Read the model definition and answer for the solid it produces. Units are mm, in the model's axes. A direction names the side the tool comes from. Coordinates: 2 decimals unless noted, no trailing zeros. Loops run counter-clockwise (first coordinate to the right, second up) from the corner with the lowest first, then second, coordinate; pieces in that order, holes last.
from build123d import *

# Parameters (mm, degrees)
PAD_DEPTH       = 8
SKETCH001_R     = 5.2
SKETCH001_R_2   = 1.75
POCKET_DEPTH    = 8.001
SKETCH002_W     = 60
SKETCH002_H     = 8
PAD001_DEPTH    = 14
SKETCH003_R     = 2.8
POCKET001_DEPTH = 30.001
FILLET_R        = 23
FILLET001_R     = 5
CHAMFER_SIZE    = 1
FILLET002_R     = 2


with BuildPart() as part:
    # Sketch → Pad (new body)
    with BuildSketch(Plane.XY):
        Polygon((-30, 0), (-30, 10), (-10, 30), (10, 30), (30, 10), (30, 0), align=None)
    extrude(amount=PAD_DEPTH)

    # Sketch001 → Pocket (cut, through all)
    with BuildSketch(Plane.XY.offset(8)):
        with Locations((0, 16)):
            Circle(SKETCH001_R)
        with Locations((-8, 16)):
            Circle(SKETCH001_R_2)
        with Locations((8, 16)):
            Circle(SKETCH001_R_2)
    extrude(amount=-POCKET_DEPTH, mode=Mode.SUBTRACT)

    # Sketch002 → Pad001 (new body)
    with BuildSketch(Plane.XY.offset(8)):
        with Locations((0, 4)):
            Rectangle(SKETCH002_W, SKETCH002_H)
    extrude(amount=PAD001_DEPTH)

    # Sketch003 → Pocket001 (cut, through all)
    with BuildSketch(Plane.XZ):
        with Locations((-21, 15)):
            Circle(SKETCH003_R)
        with Locations((21, 15)):
            Circle(SKETCH003_R)
    extrude(amount=-POCKET001_DEPTH, mode=Mode.SUBTRACT)

    # Fillet
    fillet_edges = [part.edges().sort_by_distance(p)[0] for p in [
        (10, 30, 4),
        (-10, 30, 4),
    ]]
    fillet(fillet_edges, radius=FILLET_R)

    # Fillet001
    fillet001_edges = [part.edges().sort_by_distance(p)[0] for p in [
        (30, 10, 4),
        (-30, 10, 4),
    ]]
    fillet(fillet001_edges, radius=FILLET001_R)

    # Chamfer
    chamfer_edges = [part.edges().sort_by_distance(p)[0] for p in [
        (0, 0, 0),
    ]]
    chamfer(chamfer_edges, length=CHAMFER_SIZE)

    # Fillet002
    fillet002_edges = [part.edges().sort_by_distance(p)[0] for p in [
        (30, 3.964466, 22),
        (-30, 3.964466, 22),
    ]]
    fillet(fillet002_edges, radius=FILLET002_R)


solid = part.part
Q1. Flat-ended cylindrical pins translate along their axes: pin 1 Ø5.5 at (x, y) = (-8, 16) entering from +Z; pin 2 Ø9 at (x, z) = (-21, 15) entering from +Y; pin 3 Ø5 at (y, z) = (11.5, 9) entering from +X. Find the tip coordinate at first contact, or state that the pin passes through.
Findings below:
pin 1: stops at z = 8
pin 2: stops at y = 8
pin 3: stops at x = 29.83
Q2. A cutting plane is placed at A-A (x = 21). Give the vertices of the cut face in (y, z), then the cut area to 3 significant figures.
Findings below:
outline: (0, 1) - (1, 0) - (19, 0) - (19, 8) - (8, 8) - (8, 12.2) - (0, 12.2) - close; (0, 17.8) - (8, 17.8) - (8, 22) - (0, 22) - close
area: 219 mm2
Q3. A cutting plane is placed at B-B (y = 16). Give the vertices of the cut face in (x, z), then the cut area to 3 significant figures.
Findings below:
outline: (-24, 0) - (-9.75, 0) - (-9.75, 8) - (-24, 8) - close; (-6.25, 0) - (-5.2, 0) - (-5.2, 8) - (-6.25, 8) - close; (5.2, 0) - (6.25, 0) - (6.25, 8) - (5.2, 8) - close; (9.75, 0) - (24, 0) - (24, 8) - (9.75, 8) - close
area: 245 mm2
Q4. A cutting plane is placed at D-D (y = 2). Give the vertices of the cut face in (x, z).
Findings below:
outline: (-30, 0) - (30, 0) - (30, 20) arc R2 ccw to (28, 22) - (-28, 22) arc R2 ccw to (-30, 20) - close; hole circle Ø5.6 at (-21, 15); hole circle Ø5.6 at (21, 15)
Q5. Straight lines are drawn through the part: probe 1 along Y at (x, z) = (5, 16); probe 2 along Y at (x, z) = (8, 5). For each, find the intervals that lie inside material, in ascending order.
Findings below:
probe 1: y = 0 to 8
probe 2: y = 0 to 14.25, 17.75 to 28.73
Q6. A cutting plane is placed at C-C (z = 2.75). Give the vertices of the cut face in (x, y).
Findings below:
outline: (-30, 0) - (30, 0) - (30, 7.93) arc R5 ccw to (28.54, 11.46) - (16.74, 23.26) arc R23 ccw to (0.47, 30) - (-0.47, 30) arc R23 ccw to (-16.74, 23.26) - (-28.54, 11.46) arc R5 ccw to (-30, 7.93) - close; hole circle Ø3.5 at (-8, 16); hole circle Ø10.4 at (0, 16); hole circle Ø3.5 at (8, 16)
Q7. Determine the mould class of faces 1 (the face through (29.43, 4.02, 21.4)), 2 (the face through (-23.8, 3.9, 15.1)), 3 (the face through (23, 17, 4)) for opening direction Z: +Z half, -Z half, draft (parallel to the pull), parting line (faces both ways), or undercut.
Findings below:
face 1: +Z half
face 2: undercut
face 3: draft
Q8. Which of the six approach directions +Z, -Z, +X, -X, +Y, -Y give full straight-line access (tool end or side, diameter ignored) to faces 4 (the face through (-29.43, 4.02, 21.4)), 5 (the face through (0, 22, 8))?
Findings below:
face 4: +Z, -X, +Y, -Y
face 5: +Z, +X, -X, +Y
